Read the model definition and answer for the solid it produces. Units are mm, in the model's axes. Give positions to 0.01 mm unless a question says otherwise; leave off trailing zeros. Order: outer loops, then holes, each group sorted by start corner. A loop starts at its lowest first (then second) coordinate and runs counter-clockwise, first axis right, second up. Notation, with made-up numbers: (41, -38.5) - (96, -38.5) arc R22 ccw to (96, -1.5) - close; hole circle Ø4 at (77, 28). An arc over 180 degrees is marked (long way). Write each question's results on one line, items separated by ' | '. Start each with the question number.
Q1. Find section A-A on x = -44.5. Give the vertices of the cut face in (y, z), and give its area (3 significant figures).
Q2. Find section B-B on z = 0. Give the vertices of the cut face in (x, y).
Q3. A flat-ended cylindrical pin translates along its axis: P1, Ø3, axis at x = 0, z = 2, coming from the -Y side. Find the tip coordinate at first contact, or state that the pin passes through.
Q4. Find the intervals of material crossed by line 1 along Z through (x, y) = (44.5, 0.7), in increasing order. Write a range as from..to.
from build123d import *

# Parameters (mm, degrees)
SKETCH1_W           = 130
SKETCH1_H           = 120
BOSS_EXTRUDE1_DEPTH = 3
CUT_EXTRUDE1_START  = -4
SKETCH2_R           = 1.6
CUT_EXTRUDE1_DEPTH  = 5


with BuildPart() as part:
    # Sketch1 → Boss-Extrude1 (new body)
    with BuildSketch(Plane(origin=(0, 0, 0), x_dir=(1, 0, 0), z_dir=(0, 1, 0))):
        Rectangle(SKETCH1_W, SKETCH1_H)
    extrude(amount=BOSS_EXTRUDE1_DEPTH)

    # Sketch2 → Cut-Extrude1 (cut)
    with BuildSketch(Plane(origin=(0, 3, 0), x_dir=(1, 0, 0), z_dir=(0, 1, 0)).offset(CUT_EXTRUDE1_START)):
        with Locations((44.5, 0)):
            Circle(SKETCH2_R)
    cut_extrude1 = extrude(amount=CUT_EXTRUDE1_DEPTH, mode=Mode.SUBTRACT)

    # Mirror1: Cut-Extrude1 across plane
    add(cut_extrude1.mirror(Plane(origin=(0, 0, 0), x_dir=(0, 0, 1), z_dir=(1, 0, 0))), mode=Mode.SUBTRACT)


solid = part.part
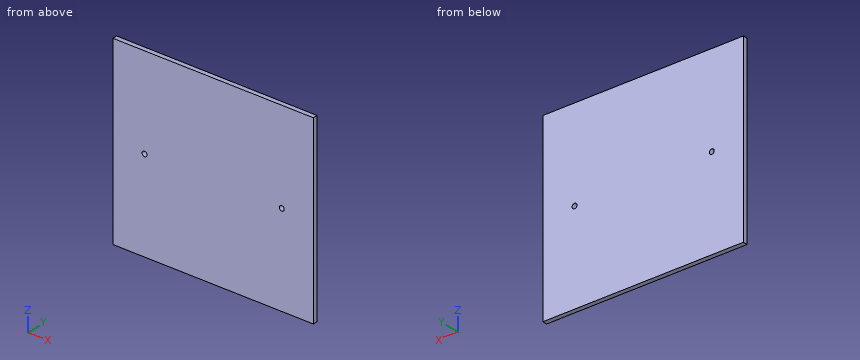
Working result:
1) outline: (0, -60) - (3, -60) - (3, -1.6) - (0, -1.6) - close; (0, 1.6) - (3, 1.6) - (3, 60) - (0, 60) - close | area: 350 mm²
2) outline: (-65, 0) - (-46.1, 0) - (-46.1, 3) - (-65, 3) - close; (-42.9, 0) - (42.9, 0) - (42.9, 3) - (-42.9, 3) - close; (46.1, 0) - (65, 0) - (65, 3) - (46.1, 3) - close
3) P1: y = 0
4) line 1: -60..-1.6, 1.6..60
